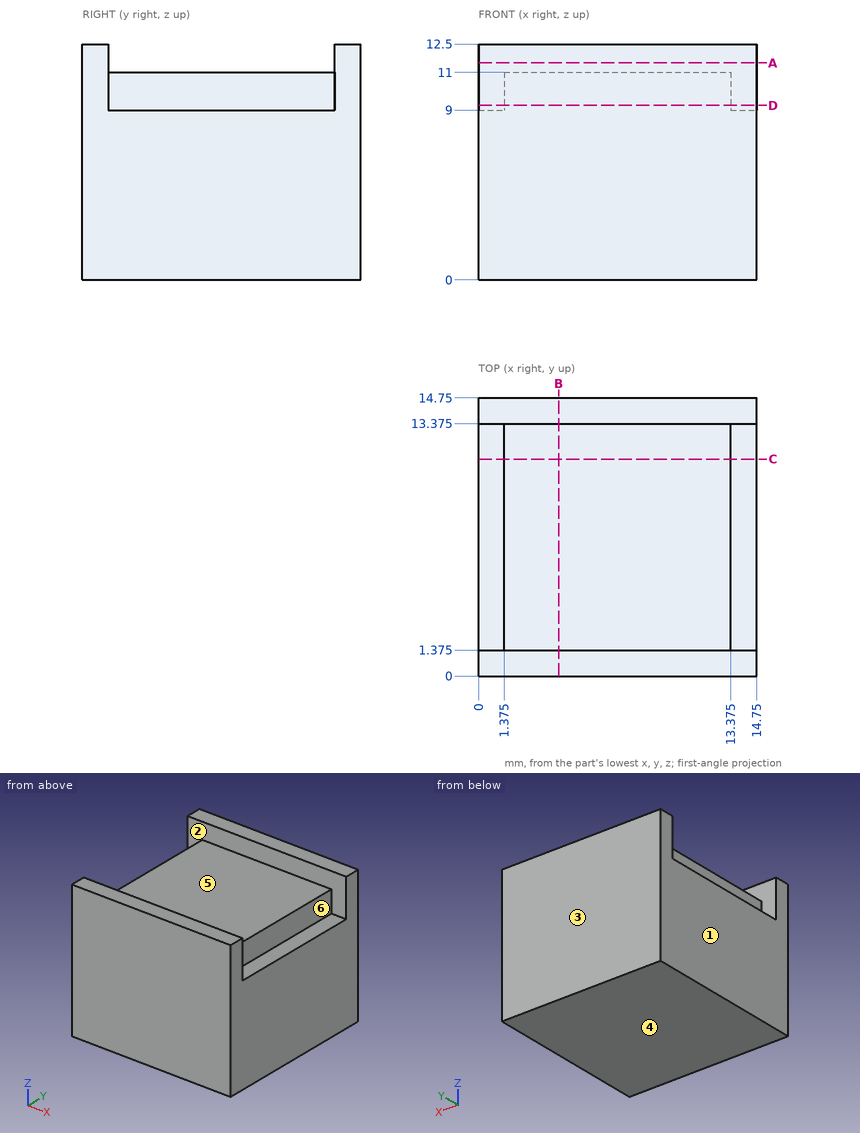
Geometry check sheet. Reference: drawing and pictorial views, mm from the part's lowest x, y, z. A direction names the side the tool comes from. Give positions to 0.01 mm unless a question says otherwise; leave off trailing zeros. Loops run counter-clockwise (first coordinate to the right, second up) from the corner with the lowest first, then second, coordinate; pieces in that order, holes last.
1. Section check D-D, the plane z = 9.25. Enter the section's corners in (x, y) (3 decimals), then the cut area to 3 significant figures.
2. Set-up check for the marked faces 4, 5 and 6: record each of +Z, -Z, +X, -X, +Y, -Y from which the full face is reachable in a straight line by a thin tool's end or side.
3. Section check B-B, the plane x = 4.25. Enter the section's corners in (y, z) (3 decimals).
4. Section check C-C, the plane y = 11.5. Enter the section's corners in (x, z) (3 decimals), then the cut area to 3 significant figures.
5. Go/stop test with flat-tipped pins: pin 1 Ø0.6 at (y, z) = (7.5, 9.5) entering from -X (3 decimals); pin 2 Ø0.7 at (x, y) = (0.5, 4.5) entering from +Z; pin 3 Ø2 at (y, z) = (7.5, 10.5) entering from +X (3 decimals). Record where each tip stops, or that it passes through.
6. Section check A-A, the plane z = 11.5. Enter the section's corners in (x, y) (3 decimals), then the cut area to 3 significant figures.
7. Thickness scan on line 1 (Z direction, x = 13.5, y = 9.5); line 2 (Z direction, x = 6.5, y = 3); line 3 (X direction, y = 11.5, z = 10) (3 decimals). Record the ranges inside material, lowest first.
8. Mould release check, pull along Y, two halves, no side actions. Record for the marked faces 1, 2 and 3: released by +Y, released by -Y, zero draft, split by the parting line, or undercut.
Geometry says:
1. outline: (0, 0) - (14.75, 0) - (14.75, 1.375) - (13.375, 1.375) - (13.375, 13.375) - (14.75, 13.375) - (14.75, 14.75) - (0, 14.75) - (0, 13.375) - (1.375, 13.375) - (1.375, 1.375) - (0, 1.375) - close
1. area: 185 mm2
2. face 4: -Z, +X, -X, +Y, -Y
2. face 5: +Z, +X, -X
2. face 6: +Z, +X
3. outline: (0, 0) - (14.75, 0) - (14.75, 12.5) - (13.375, 12.5) - (13.375, 11) - (1.375, 11) - (1.375, 12.5) - (0, 12.5) - close
4. outline: (0, 0) - (14.75, 0) - (14.75, 9) - (13.375, 9) - (13.375, 11) - (1.375, 11) - (1.375, 9) - (0, 9) - close
4. area: 157 mm2
5. pin 1: stops at x = 1.375
5. pin 2: stops at z = 9
5. pin 3: stops at x = 13.375
6. outline: (0, 0) - (14.75, 0) - (14.75, 1.375) - (0, 1.375) - close; (0, 13.375) - (14.75, 13.375) - (14.75, 14.75) - (0, 14.75) - close
6. area: 40.6 mm2
7. line 1: z = 0 to 9
7. line 2: z = 0 to 11
7. line 3: x = 1.375 to 13.375
8. face 1: zero draft
8. face 2: undercut
8. face 3: released by +Y
